Verification items for this drawing (mm, ordinates from the low corner). Give positions to 0.01 mm unless a question says otherwise; leave off trailing zeros. Loops run counter-clockwise (first coordinate to the right, second up) from the corner with the lowest first, then second, coordinate; pieces in that order, holes last. Notation, with made-up numbers: (62, -25.5) -> (70, -25.5) arc R17 cw to (70, -12.5) -> close; hole circle Ø2 at (-26, 68.5). An arc over 180 degrees is marked (long way). Answer in a Markdown table with one row per item. Add a question column.
Q1. Gauge pin test, flat end, axial feed: P1, Ø2, axis at x = 88, y = 0.5, coming from the -Z side. Record the tip position at first contact, or that the pin passes through.
Q2. Section check B-B on x = 112.5. Enter the section's corners in (y, z).
Q3. Material ranges on probe 1 along X at (y, z) = (1.4, 10); probe 2 along Z at (x, y) = (115, 3); probe 3 along X at (y, z) = (1.55, 227.5) (1 decimal), recorded low to high.
Q4. Section check A-A on z = 10. Enter the section's corners in (x, y).
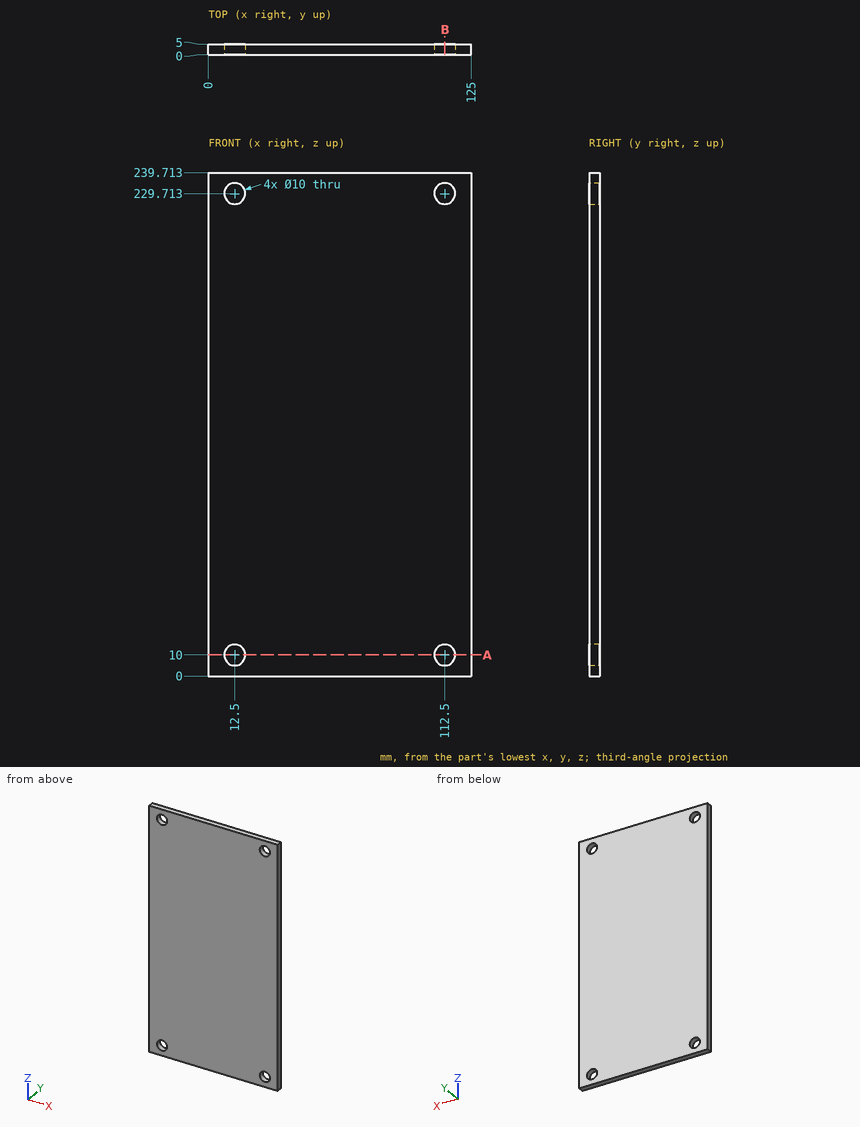
Taken from the geometry:
| question | item | result |
|---|---|---|
| 1 | P1 | stops at z = 0 |
| 2 | outline | (0, 0) -> (5, 0) -> (5, 5) -> (0, 5) -> close; (0, 15) -> (5, 15) -> (5, 224.71) -> (0, 224.71) -> close; (0, 234.71) -> (5, 234.71) -> (5, 239.71) -> (0, 239.71) -> close |
| 3 | probe 1 | x = 0 to 7.5, 17.5 to 107.5, 117.5 to 125 |
| 3 | probe 2 | z = 0 to 5.67, 14.33 to 225.38, 234.04 to 239.71 |
| 3 | probe 3 | x = 0 to 8, 17 to 108, 117 to 125 |
| 4 | outline | (0, 0) -> (7.5, 0) -> (7.5, 5) -> (0, 5) -> close; (17.5, 0) -> (107.5, 0) -> (107.5, 5) -> (17.5, 5) -> close; (117.5, 0) -> (125, 0) -> (125, 5) -> (117.5, 5) -> close |
